Part model, mm, in its own coordinate system. Face numbers are marked on the shaded views. A direction names the side the tool comes from. Give positions to 0.01 mm unless a question says otherwise; leave off trailing zeros. Order: outer loops, then holes, each group sorted by start corner. A loop starts at its lowest first (then second) coordinate and runs counter-clockwise, first axis right, second up.
1. Slice it at A-A on z = -60. List the corners of the cut face in (x, y), and give its area (3 significant figures).
2. Probe line 1 (X direction, y = 3.3, z = -20); line 2 (Z direction, x = 0, y = 1.4); line 3 (Y direction, x = 0, z = -1.4). List the from-to ranges inside material, lowest first.
3. Slice it at B-B on x = 0. List the corners of the cut face in (y, z), and give its area (3 significant figures).
4. Which spindle directions (+Z, -Z, +X, -X, +Y, -Y) get a long thin tool onto all of the face, cutting with end or side? Do the marked faces 1 and 2. Say none if no direction does.
5. Slice it at D-D on x = -7. List the corners of the cut face in (y, z).
6. Slice it at C-C on y = 20. List the corners of the cut face in (x, z).
7. Drop flat-ended pins along their axis: pin 1 Ø6.5 at (x, y) = (0, 20) entering from -Z; pin 2 Ø8 at (x, y) = (-13.5, 15) entering from +Z; pin 3 Ø6 at (x, z) = (9.5, -13.5) entering from +Y. Give the stop position or say it passes through.
from build123d import *

# Parameters (mm, degrees)
BOSS_EXTRUDE1_DEPTH = 18
SKETCH2_R           = 5.1
SKETCH2_R_2         = 4.15
CUT_EXTRUDE1_DEPTH  = 7
SKETCH3_R           = 4.15
CUT_EXTRUDE2_DEPTH  = 7
FILLET1_R           = 5
CHAMFER1_SIZE       = 0.75


with BuildPart() as part:
    # Sketch1 → Boss-Extrude1 (new body, symmetric)
    with BuildSketch(Plane(origin=(0, 0, 0), x_dir=(0, 0, -1), z_dir=(1, 0, 0))):
        Polygon((0, 40), (0, 0), (80, 0), (80, 6), (6, 6), (6, 40), align=None)
    extrude(amount=BOSS_EXTRUDE1_DEPTH, both=True)

    # Sketch2 → Cut-Extrude1 (cut, through all)
    with BuildSketch(Plane(origin=(0, 6, 0), x_dir=(1, 0, 0), z_dir=(0, 1, 0))):
        with Locations((0, 60)):
            Circle(SKETCH2_R)
        with Locations((0, 20)):
            Circle(SKETCH2_R_2)
    extrude(amount=-CUT_EXTRUDE1_DEPTH, mode=Mode.SUBTRACT)

    # Sketch3 → Cut-Extrude2 (cut, through all)
    with BuildSketch(Plane(origin=(0, 0, -6), x_dir=(-1, 0, 0), z_dir=(0, 0, -1))):
        with Locations((0, 20)):
            Circle(SKETCH3_R)
    extrude(amount=-CUT_EXTRUDE2_DEPTH, mode=Mode.SUBTRACT)

    # Fillet1
    fillet1_edges = [part.edges().sort_by_distance(p)[0] for p in [
        (0, 40, -6),
        (0, 6, -6),
        (0, 6, -80),
    ]]
    fillet(fillet1_edges, radius=FILLET1_R)

    # Chamfer1
    chamfer1_edges = [part.edges().sort_by_distance(p)[0] for p in [
        (-5.1, 0, -60),
        (-5.1, 6, -60),
    ]]
    chamfer(chamfer1_edges, length=CHAMFER1_SIZE)


solid = part.part
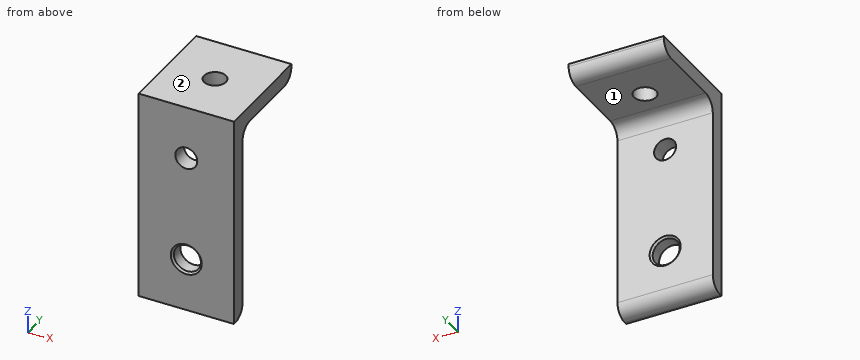
Data:
1. outline: (-18, 0) - (-5.85, 0) - (-5.1, 0.75) - (-5.1, 5.25) - (-5.85, 6) - (-18, 6) - close; (5.1, 0.75) - (5.85, 0) - (18, 0) - (18, 6) - (5.85, 6) - (5.1, 5.25) - close
1. area: 154 mm2
2. line 1: x = -18 to -4.15, 4.15 to 18
2. line 2: z = -79.98 to -65.1, -54.9 to -24.15, -15.85 to 0
2. line 3: y = 0 to 15.85, 24.15 to 39.98
3. outline: (0, -80) - (1, -80) arc R5 ccw to (6, -75) - (6, -65.85) - (5.25, -65.1) - (0.75, -65.1) - (0, -65.85) - close; (0, -54.15) - (0.75, -54.9) - (5.25, -54.9) - (6, -54.15) - (6, -24.15) - (0, -24.15) - close; (0, -15.85) - (6, -15.85) - (6, -11) arc R5 cw to (11, -6) - (15.85, -6) - (15.85, 0) - (0, 0) - close; (24.15, -6) - (35, -6) arc R5 ccw to (40, -1) - (40, 0) - (24.15, 0) - close
3. area: 517 mm2
4. face 1: -Z, +X, -X, +Y
4. face 2: +Z, +X, -X, +Y, -Y
5. outline: (0, -80) - (1, -80) arc R5 ccw to (6, -75) - (6, -11) arc R5 cw to (11, -6) - (35, -6) arc R5 ccw to (40, -1) - (40, 0) - (0, 0) - close
6. outline: (-18, -6) - (-4.15, -6) - (-4.15, 0) - (-18, 0) - close; (4.15, -6) - (18, -6) - (18, 0) - (4.15, 0) - close
7. pin 1: passes through
7. pin 2: stops at z = 0
7. pin 3: stops at y = 6.03
